```python
from build123d import *

# Parameters (mm, degrees)
BOSS_EXTRUDE1_DEPTH = 3
SKETCH2_W           = 5
SKETCH2_H           = 20
CUT_EXTRUDE1_DEPTH  = 2


with BuildPart() as part:
    # Sketch1 → Boss-Extrude1 (new body)
    with BuildSketch(Plane(origin=(0, 0, 0), x_dir=(1, 0, 0), z_dir=(0, 1, 0))):
        Polygon((0, 4), (0, 0), (44, 0), (44, 4), (42, 4), (42, 8), (44, 8), (44, 12), (42, 12), (42, 16), (44, 16), (44, 20), (0, 20), (0, 16), (2, 16), (2, 12), (0, 12), (0, 8), (2, 8), (2, 4), align=None)
    extrude(amount=BOSS_EXTRUDE1_DEPTH)

    # Sketch2 → Cut-Extrude1 (cut)
    with BuildSketch(Plane(origin=(0, 3, 0), x_dir=(1, 0, 0), z_dir=(0, 1, 0))):
        with Locations((41.5, 10)):
            Rectangle(SKETCH2_W, SKETCH2_H)
        with Locations((2.5, 10)):
            Rectangle(SKETCH2_W, SKETCH2_H)
    extrude(amount=-CUT_EXTRUDE1_DEPTH, mode=Mode.SUBTRACT)


solid = part.part
```
CAD build for the part. Positions are in the model's coordinates, mm. A direction names the side the tool comes from. Coordinates: 2 decimals unless noted, no trailing zeros. Order: outer loops, then holes, each group sorted by start corner. A loop starts at its lowest first (then second) coordinate and runs counter-clockwise, first axis right, second up.
(1) Which spindle directions (+Z, -Z, +X, -X, +Y, -Y) get a long thin tool onto all of the face, cutting with end or side? Do faces 1 (the face through (39, 2, -10)), 2 (the face through (42, 0.5, -14)), 3 (the face through (5, 2, -10)), 4 (the face through (2, 0.5, -14)), 5 (the face through (44, 0.5, -2)). Say none if no direction does.
Solution:
face 1: +Z, -Z, +X, +Y
face 2: +X, +Y, -Y
face 3: +Z, -Z, -X, +Y
face 4: -X, +Y, -Y
face 5: +Z, -Z, +X, +Y, -Y
(2) Drill centre lines: L1, parallel to X at y = 2.7, z = -7; L2, parallel to Y at x = 3, z = -15; L3, parallel to X at y = 0.7, z = -12.75. Where is each one in solid material? Low to high.
Solution:
L1: x = 5 to 39
L2: y = 0 to 1
L3: x = 2 to 42
(3) Saw through at B-B, the plane y = 1.65. Write the cut outline in (x, z), and give its area (3 significant figures).
Solution:
outline: (5, -20) - (39, -20) - (39, 0) - (5, 0) - close
area: 680 mm2
(4) Saw through at A-A, the plane z = -10.5. Write the cut outline in (x, y), and give its area (3 significant figures).
Solution:
outline: (0, 0) - (44, 0) - (44, 1) - (39, 1) - (39, 3) - (5, 3) - (5, 1) - (0, 1) - close
area: 112 mm2
(5) Mould opens along Z. For faces 6 (the face through (1, 0.5, -4)), 7 (the face through (0, 0.5, -2)), 8 (the face through (43, 0.5, -12)) say: released by +Z, released by -Z, zero draft, split by the parting line, or undercut.
Solution:
face 6: undercut
face 7: zero draft
face 8: undercut
(6) Pin check, flat tips, straight feed: pin 1 Ø3 at (x, z) = (23, -3) entering from -Y; pin 2 Ø1 at (y, z) = (2.5, -14) entering from +X; pin 3 Ø0.8 at (y, z) = (0.5, -6.5) entering from -X; pin 4 Ø0.8 at (y, z) = (0.5, -15) entering from +X. Stop position of each tip, or through.
Solution:
pin 1: stops at y = 0
pin 2: stops at x = 39
pin 3: stops at x = 2
pin 4: stops at x = 42
(7) Saw through at C-C, the plane x = 39.5. Write the cut outline in (y, z).
Solution:
outline: (0, -20) - (1, -20) - (1, 0) - (0, 0) - close
(8) Saw through at D-D, the plane z = -4.5. Write the cut outline in (x, y), and give its area (3 significant figures).
Solution:
outline: (2, 0) - (42, 0) - (42, 1) - (39, 1) - (39, 3) - (5, 3) - (5, 1) - (2, 1) - close
area: 108 mm2
